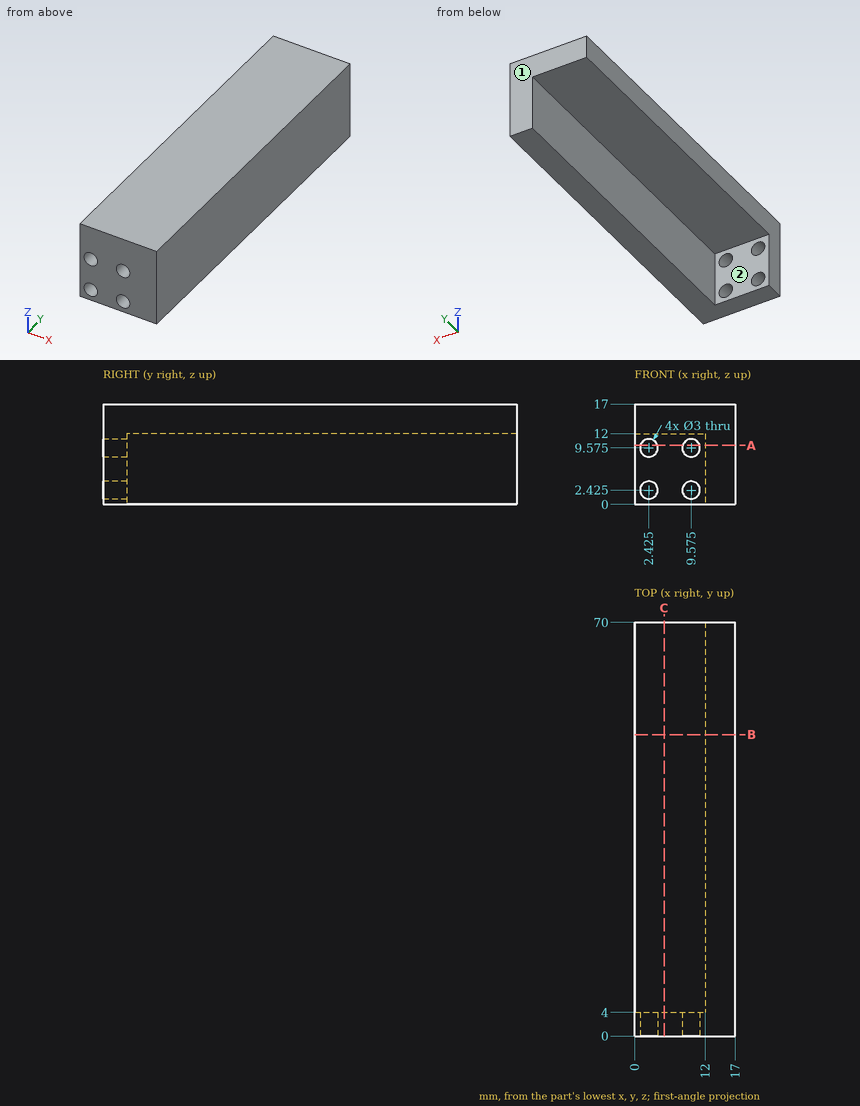
Answer from the drawing. Dimensions are ordinates in mm from the lowest x, y and z of the part. A direction names the side the tool comes from. Coordinates: 2 decimals unless noted, no trailing zeros. Order: outer loops, then holes, each group sorted by start corner. A loop starts at its lowest first (then second) coordinate and runs counter-clockwise, first axis right, second up. Notation, with made-up numbers: M 29.5,-20 L 78.5,-20 A28 ccw 78.5,8 Z; hole C -12.5,34 d10. An arc over 180 degrees is marked long. Put each result on its own line as item: value. Start each with the question number.
Item 1: Section A-A, the plane z = 10 is taken. Determine the outline of the cut face in (x, y).
Item 2: Given pin 1 Ø4 at (x, z) = (10.5, 11.5) entering from -Y; pin 2 Ø3 at (y, z) = (23.5, 5.5) entering from -X; pin 3 Ø9.5 at (x, z) = (4.5, 3) entering from +Y; pin 4 Ø4 at (x, y) = (9, 61.5) entering from -Z, each flat-ended and moving along its own axis, determine where each tip first touches the part or whether it passes through.
Item 3: For the marked faces 1 and 2, determine the directions among +Z, -Z, +X, -X, +Y, -Y from which every point of the face is accessible in a straight line to the end or side of a thin tool.
Item 4: Section B-B, the plane y = 51 is taken. Determine the outline of the cut face in (x, z), plus the area to 3 significant figures.
Item 5: Consider probe 1 along Z at (x, y) = (8.75, 48); probe 2 along Y at (x, z) = (5.25, 8.75). Determine where each line is inside the solid, lowest interval first. Write a range as [from, to].
Item 6: Section C-C, the plane x = 5 is taken. Determine the outline of the cut face in (y, z).
Computed:
1. outline: M 0,0 L 0.99,0 L 0.99,4 L 0,4 Z; M 3.86,0 L 8.14,0 L 8.14,4 L 3.86,4 Z; M 11.01,0 L 17,0 L 17,70 L 12,70 L 12,4 L 11.01,4 Z
2. pin 1: stops at y = 0
2. pin 2: stops at x = 12
2. pin 3: stops at y = 4
2. pin 4: stops at z = 12
3. face 1: +Z, -Z, +X, -X, +Y
3. face 2: -Z, -X, +Y
4. outline: M 0,12 L 12,12 L 12,0 L 17,0 L 17,17 L 0,17 Z
4. area: 145 mm2
5. probe 1: z = [12, 17]
5. probe 2: y = [0, 4]
6. outline: M 0,0 L 4,0 L 4,12 L 70,12 L 70,17 L 0,17 Z
